The listing builds one solid part. Answer for the finished solid, in the listing's coordinates (mm). Face numbers are marked on the shaded views. A direction names the side the tool comes from. Round coordinates to 2 decimals unless told otherwise and drop trailing zeros. Write each loop counter-clockwise with the first axis right and the second up, starting at its lowest first coordinate (ties: lowest second). Pieces come first, ordered by that corner, then holes. Notation, with made-up numbers: M -30,30.25 L 9,30.25 A30 cw 9,53.25 Z; hole C 64,8 d10. An arc over 180 degrees is marked long. Answer as CSV lines item,"result". Start each with the question number.
from build123d import *

# Parameters (mm, degrees)
BOSS_EXTRUDE1_DEPTH = 1.25
FILLET1_R           = 1.25


with BuildPart() as part:
    # Sketch1 → Boss-Extrude1 (new, symmetric)
    with BuildSketch(Plane.XY):
        Polygon((-5, 7.5), (-5, -7.5), (-2.5, -7.5), (-2.5, 0), (2.5, 0), (2.5, -7.5), (5, -7.5), (5, 7.5), align=None)
    extrude(amount=BOSS_EXTRUDE1_DEPTH, both=True)

    # Fillet1
    fillet1_edges = [part.edges().sort_by_distance(p)[0] for p in [
        (-2.5, -7.5, 0),
        (-5, -7.5, 0),
        (-5, 7.5, 0),
        (5, 7.5, 0),
        (2.5, -7.5, 0),
        (5, -7.5, 0),
    ]]
    fillet(fillet1_edges, radius=FILLET1_R - 0.0001)  # a hair under: the kernel refuses the full size


solid = part.part
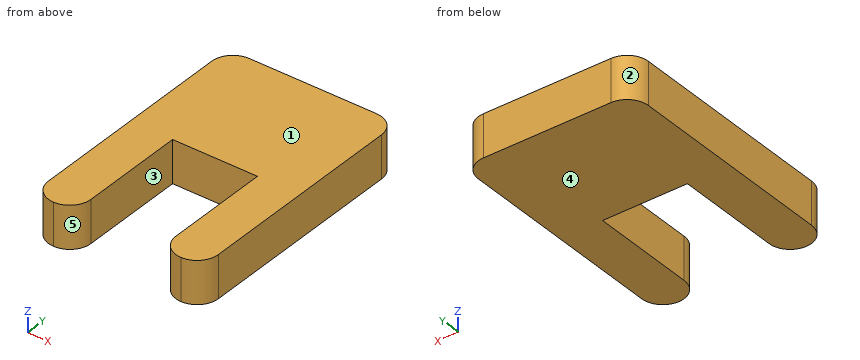
Q1. The mould has two halves that part along X. Classify the marked faces 1, 2 and 3: +X half, -X half, draft (parallel to the pull), parting line (faces both ways), or undercut.
Q2. Find section C-C (x = 0). Determine the outline of the cut face in (y, z), plus the area to 4 significant figures.
Q3. Straight lines are drawn through the part: L1, parallel to X at y = -3.25, z = 0.9; L2, parallel to Y at x = 1.75, z = 0.2; L3, parallel to X at y = 6.75, z = -0.5. For each, find the intervals that lie inside material, in ascending order.
Q4. Find section A-A (y = -3). Determine the outline of the cut face in (x, z).
Q5. Each of these flat-tipped pins is pushed along its axis until it touches: P1, Ø0.8, axis at x = -0.5, z = 0.5, coming from the -Y side; P2, Ø1, axis at x = 2.5, z = 1, coming from the -Y side; P3, Ø2, axis at x = 2, y = -1.5, coming from the +Z side; P4, Ø1, axis at x = 1, y = -3, coming from the -Z side. Where does it stop, or does it pass through?
Q6. For the marked faces 4 and 5, determine the directions among +Z, -Z, +X, -X, +Y, -Y from which every point of the face is accessible in a straight line to the end or side of a thin tool.
Q7. Find section D-D (x = -3). Determine the outline of the cut face in (y, z), plus the area to 3 significant figures.
Reported:
1,face 1,"draft"
1,face 2,"-X half"
1,face 3,"undercut"
2,outline,"M 0,-1.25 L 7.5,-1.25 L 7.5,1.25 L 0,1.25 Z"
2,area,"18.75 mm2"
3,L1,"x = -5 to -2.5, 2.5 to 5"
3,L2,"y = 0 to 7.5"
3,L3,"x = -4.9 to 4.9"
4,outline,"M -5,-1.25 L -2.5,-1.25 L -2.5,1.25 L -5,1.25 Z; M 2.5,-1.25 L 5,-1.25 L 5,1.25 L 2.5,1.25 Z"
5,P1,"stops at y = 0"
5,P2,"stops at y = -7.25"
5,P3,"stops at z = 1.25"
5,P4,"passes through"
6,face 4,"-Z, +X, -X, +Y, -Y"
6,face 5,"+Z, -Z, -Y"
7,outline,"M -7.25,-1.25 L 7.5,-1.25 L 7.5,1.25 L -7.25,1.25 Z"
7,area,"36.9 mm2"
